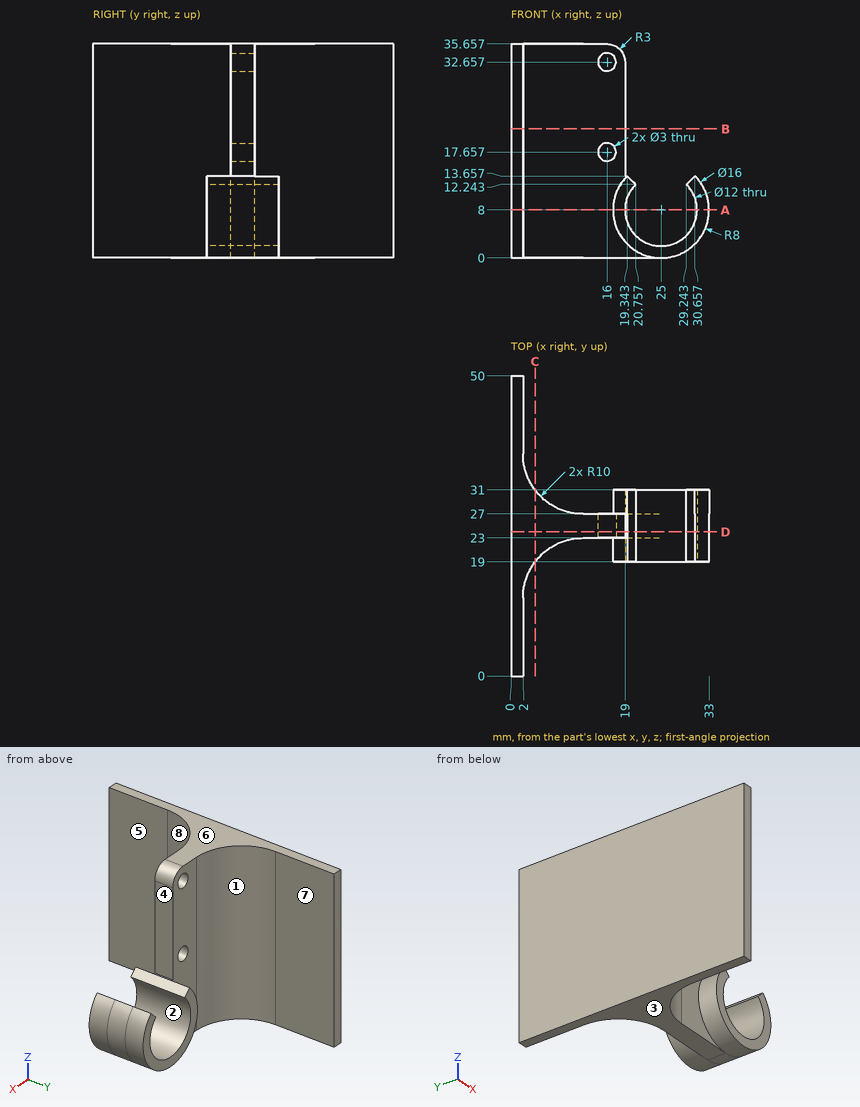
Design review of the part shown in the three views and the two pictorial views. Dimensions are in mm from the part's minimum x, y and z. A direction names the side the tool comes from. Give positions to 0.01 mm unless a question says otherwise; leave off trailing zeros. Loops run counter-clockwise (first coordinate to the right, second up) from the corner with the lowest first, then second, coordinate; pieces in that order, holes last. Notation, with made-up numbers: (-15.5, 87) - (-4.5, 87) arc R23 cw to (-4.5, 120) - close; hole circle Ø9 at (-1, 88.25). An arc over 180 degrees is marked (long way). Write item = value, one per line.
1) Clearance check with flat-ended pins moving along their axes: pin 1 Ø11 at (x, z) = (28.5, 7.5) entering from +Y; pin 2 Ø5 at (x, z) = (16, 32.66) entering from -Y; pin 3 Ø12 at (y, z) = (17.5, 9.5) entering from +X; pin 4 Ø2 at (y, z) = (24, 19.5) entering from +X. State where each tip first meets the part, or that it passes through.
Result sheet:
pin_1 = 31
pin_2 = 23
pin_3 = 33
pin_4 = 19
2) Take a section at A-A on z = 8. State the section outline as (x, y) points, and give its area (3 significant figures).
Result sheet:
outline = (0, 0) - (2, 0) - (2, 13) arc R10 cw to (12, 23) - (17, 23) - (17, 19) - (19, 19) - (19, 31) - (17, 31) - (17, 27) - (12, 27) arc R10 cw to (2, 37) - (2, 50) - (0, 50) - close; (31, 19) - (33, 19) - (33, 31) - (31, 31) - close
area = 251 mm2
3) Take a section at C-C on x = 4. State the section outline as (y, z) points, and give its area (3 significant figures).
Result sheet:
outline = (19, 0) - (31, 0) - (31, 35.66) - (19, 35.66) - close
area = 428 mm2
4) Draft analysis for pull direction X (two halves, no side actions). For the marked faces 1, 2, 3 and 4, state which applies: +X half, -X half, draft (parallel to the pull), parting line (faces both ways), or undercut.
Result sheet:
face_1 = undercut
face_2 = undercut
face_3 = draft
face_4 = +X half
5) Take a section at B-B on z = 21.5. State the section outline as (x, y) points.
Result sheet:
outline = (0, 0) - (2, 0) - (2, 13) arc R10 cw to (12, 23) - (19, 23) - (19, 27) - (12, 27) arc R10 cw to (2, 37) - (2, 50) - (0, 50) - close
6) Tool access review of the marked faces 5, 6, 7 and 8: name each direction out of +Z, -Z, +X, -X, +Y, -Y from which nothing blocks a thin tool from reaching the whole face with its end or side.
Result sheet:
face_5 = +Z, -Z, +X, -Y
face_6 = +Z, +X, -X, +Y, -Y
face_7 = +Z, -Z, +X, +Y
face_8 = +Z, -Z, -Y
7) Take a section at D-D on y = 24. State the section outline as (x, z) points.
Result sheet:
outline = (0, 0) - (25, 0) arc R8 ccw to (30.66, 13.66) - (29.24, 12.24) arc R6 cw (long way) to (20.76, 12.24) - (19.34, 13.66) - (19, 13.66) - (19, 32.66) arc R3 ccw to (16, 35.66) - (0, 35.66) - close; hole circle Ø3 at (16, 17.66); hole circle Ø3 at (16, 32.66)
8) To check wall thickness, follow line 1 (Z direction, x = 16, y = 24.95); line 2 (X direction, y = 26.75, z = 8); line 3 (Y direction, x = 11.5, z = 26). State the ranges of each line that lie inside material, in increasing order.
Result sheet:
line_1 = 0 to 16.16, 19.16 to 31.16, 34.16 to 35.66
line_2 = 0 to 19, 31 to 33
line_3 = 22.99 to 27.01
